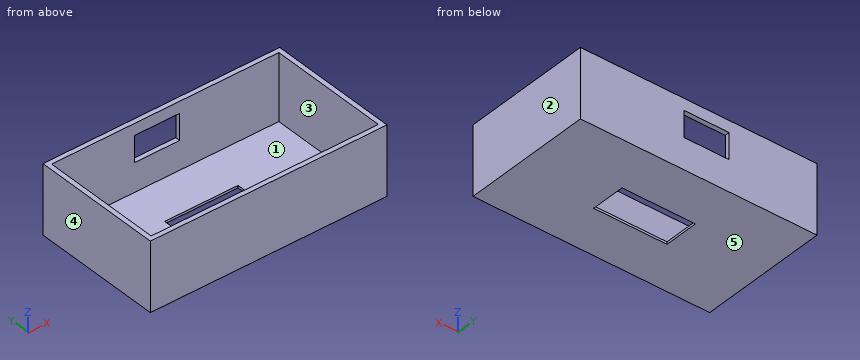
Autodesk Fusion 360 part; units mm, degrees
sketch "Sketch1" plane through (0, 0, 0) normal (0, 0, 1) x (1, 0, 0)
  line L0 (0, 0) -> (100, 0)
  line L1 (100, 0) -> (100, 55)
  line L2 (100, 55) -> (0, 55)
  line L3 (0, 55) -> (0, 0)
  line L4 (2, 2) -> (98, 2)
  line L5 (98, 2) -> (98, 53)
  line L6 (98, 53) -> (2, 53)
  line L7 (2, 53) -> (2, 2)
  line L8 (34.5, 34.5) -> (65.5, 34.5)
  line L9 (65.5, 34.5) -> (65.5, 20)
  line L10 (65.5, 20) -> (34.5, 20)
  line L11 (34.5, 20) -> (34.5, 34.5)
  dimension "d1" = -2
  dimension "d12" = 31
  dimension "d13" = 14.5
  dimension "d14" = 96
  dimension "d15" = 32.5
  dimension "d16" = 51
  dimension "d17" = 55
  dimension "d18" = 20
extrude "Extrude1" add sketch "Sketch1" along normal blind 1 contours L4 L5 L6 L7
extrude "Extrude2" add sketch "Sketch1" along normal blind 4 contours L0 L1 L2 L3
extrude "Extrude3" add 1 faces at (34, 0.6667, 4) along direction (0, 0, 1) blind 50
sketch "Sketch2" plane through (0, 55, 0) normal (0, 1, 0) x (-1, 0, 0)
  line L0 (-100, 0) -> (0, 0)
  line L1 (0, 0) -> (0, 54)
  line L2 (0, 54) -> (-100, 54)
  line L3 (-100, 54) -> (-100, 0)
  line L4 (-56.0994, 24.0994) -> (-37.0994, 24.0994)
  line L5 (-37.0994, 24.0994) -> (-37.0994, 13.0994)
  line L6 (-37.0994, 13.0994) -> (-56.0994, 13.0994)
  line L7 (-56.0994, 13.0994) -> (-56.0994, 24.0994)
  dimension "d8" = 19
  dimension "d9" = 11
extrude "Extrude4" cut sketch "Sketch2" against normal blind 15 contours L4 L5 L6 L7
extrude "Extrude5" cut 1 faces at (34, 0.6667, 54) along direction (0, 0, -1) blind 25
Can you work these out from the model? Positions are in its coordinate system, mm. Face numbers are marked on the shaded views. A direction names the side the tool comes from. Coordinates: 2 decimals unless noted, no trailing zeros. Loops run counter-clockwise (first coordinate to the right, second up) from the corner with the lowest first, then second, coordinate; pieces in that order, holes last.
1) Thinking about a two-plate mould opening in X: for the marked faces 3, 4 and 5, which applies, pulls with the +X half, pulls with the -X half, needs draft (parallel to the pull), parting line crosses it, or undercut?
2) Imagine slicing it at C-C on y = 12.5. List the corners of the cut face in (x, z) for me.
3) Which directions (+Z, -Z, +X, -X, +Y, -Y) give clear straight access to the entire face, cutting with the end or side of a thin tool? Please do the marked faces 1 and 2.
4) Imagine slicing it at A-A on y = 29. List the corners of the cut face in (x, z) for me.
5) Imagine slicing it at D-D on x = 89. List the corners of the cut face in (y, z) for me.
6) Imagine slicing it at B-B on z = 10.5. List the corners of the cut face in (x, y) for me, plus the area to 3 significant figures.
7) I need wall thicknesses on probe 1 along X at (y, z) = (12.5, 9); probe 2 along Y at (x, z) = (60.5, 26); probe 3 along Z at (x, y) = (71, 39). Which ranges of each line are inside material? Lowest first, please.
8) For pin 1 (5 mm diameter, centred on x = 82, y = 33, fed in from +Z), with a flat end and sliding along its axis, tell me the tip position at first contact or that it passes through.
Completed:
1. face 3: undercut
1. face 4: pulls with the -X half
1. face 5: needs draft
2. outline: (0, 0) - (100, 0) - (100, 29) - (98, 29) - (98, 1) - (2, 1) - (2, 29) - (0, 29) - close
3. face 1: +Z
3. face 2: +Z, -Z, +X, +Y, -Y
4. outline: (0, 0) - (34.5, 0) - (34.5, 1) - (2, 1) - (2, 29) - (0, 29) - close; (65.5, 0) - (100, 0) - (100, 29) - (98, 29) - (98, 1) - (65.5, 1) - close
5. outline: (0, 0) - (55, 0) - (55, 29) - (53, 29) - (53, 1) - (2, 1) - (2, 29) - (0, 29) - close
6. outline: (0, 0) - (100, 0) - (100, 55) - (0, 55) - close; hole (2, 2) - (98, 2) - (98, 53) - (2, 53) - close
6. area: 604 mm2
7. probe 1: x = 0 to 2, 98 to 100
7. probe 2: y = 0 to 2, 53 to 55
7. probe 3: z = 0 to 1
8. pin 1: stops at z = 1
